Check sheet for the modelled part. Datum: model origin and axes. Units: mm. A direction names the side the tool comes from. Give positions to 0.01 mm unless a question says otherwise; leave off trailing zeros. Write each loop counter-clockwise with the first axis right and the second up, starting at its lowest first coordinate (ties: lowest second). Pieces come first, ordered by that corner, then holes. Notation, with made-up numbers: M -18,34 L 16,34 A6 cw 16,44 Z; hole C 29,-11.75 d6. An arc over 180 degrees is marked long. Write item = value, one per line. Start each with the question number.
1) Sectioned sample at C-C, the plane y = 1. Record the cut outline in (x, z) (3 decimals).
2) Gauge pin test, flat ends, axial feed: pin 1 (3.5 mm diameter, centred on x = 0, z = 0, fed in from -Y); pin 2 (2 mm diameter, centred on y = -4.5, z = -3.5, fed in from -X); pin 3 (1.6 mm diameter, centred on x = -11.5, z = 11.5, fed in from -Y); pin 4 (1.2 mm diameter, centred on x = -11.5, z = -11.5, fed in from +Y). Record the tip position at first contact, or that the pin passes through.
3) Sectioned sample at A-A, the plane y = 31. Record the cut outline in (x, z).
4) Draft check along X on faces 5 (the face through (6, 47, 16)), 6 (the face through (-2.003, 21.496, -0.631)), 7 (the face through (-3, 50, 3)), 8 (the face through (0, 25, 14.1)). Enter one of: pulls with the +X half, pulls with the -X half, needs draft (parallel to the pull), parting line crosses it, or undercut.
5) Scan lines: L1, parallel to Z at x = 0, y = 50.2; L2, parallel to Z at x = 0, y = 24.5; L3, parallel to Z at x = -11.5, y = 7.75 (3 decimals). Record each from-to range of solid material in increasing order.
6) Set-up check for faces 1 (the face through (-12.26, 7.6, -12.19)), 2 (the face through (11, 48, 11)), 3 (the face through (6, 51, 0)), 4 (the face through (-13, 49, -8.5)): record each of +Z, -Z, +X, -X, +Y, -Y from which the full face is reachable in a straight line by a thin tool's end or side.
from build123d import *

# Parameters (mm, degrees)
SKETCH1_W               = 28.2
SKETCH1_H               = 28.2
BOSS_EXTRUDE1_DEPTH     = 51
SKETCH2_R               = 11
BOSS_EXTRUDE2_DEPTH     = 2
M2_5_TAPPED_HOLE1_D     = 2.05
M2_5_TAPPED_HOLE1_DEPTH = 15
M2_5_TAPPED_HOLE1_TIP   = 0.615882135
FILLET1_R               = 3
SKETCH6_R               = 4
BOSS_EXTRUDE3_DEPTH     = 14
SKETCH7_R               = 4
BOSS_EXTRUDE4_DEPTH     = 7
M5_TAPPED_HOLE1_D       = 4.2
CHAMFER1_SIZE           = 0.2
SKETCH10_R              = 4.5
SKETCH10_R_2            = 4
CUT_EXTRUDE1_DEPTH      = 1
SKETCH11_W              = 12
SKETCH11_H              = 4
BOSS_EXTRUDE5_DEPTH     = 3
CUT_EXTRUDE2_DEPTH      = 3
CIRPATTERN1_COUNT       = 4
FILLET2_R               = 0.5


with BuildPart() as part:
    # Sketch1 → Boss-Extrude1 (new body)
    with BuildSketch(Plane(origin=(0, 0, 0), x_dir=(1, 0, 0), z_dir=(0, 1, 0))):
        Rectangle(SKETCH1_W, SKETCH1_H)
    extrude(amount=BOSS_EXTRUDE1_DEPTH)

    # Sketch2 → Boss-Extrude2 (add)
    with BuildSketch(Plane.XZ):
        Circle(SKETCH2_R)
    extrude(amount=BOSS_EXTRUDE2_DEPTH)

    # M2.5 Tapped Hole1
    with Locations(Plane(origin=(0, 0, 0), x_dir=(-1, 0, 0), z_dir=(0, -1, 0))):
        with Locations((11.5, -11.5), (-11.5, -11.5), (-11.5, 11.5), (11.5, 11.5)):
            Hole(M2_5_TAPPED_HOLE1_D / 2, depth=M2_5_TAPPED_HOLE1_DEPTH)
            with Locations((0, 0, -(M2_5_TAPPED_HOLE1_DEPTH + M2_5_TAPPED_HOLE1_TIP / 2))):  # 118° drill point
                Cone(0, M2_5_TAPPED_HOLE1_D / 2, M2_5_TAPPED_HOLE1_TIP, mode=Mode.SUBTRACT)

    # Fillet1
    fillet1_edges = [part.edges().sort_by_distance(p)[0] for p in [
        (14.1, 25.5, 14.1),
        (-14.1, 25.5, 14.1),
        (-14.1, 25.5, -14.1),
        (14.1, 25.5, -14.1),
    ]]
    fillet(fillet1_edges, radius=FILLET1_R)

    # Sketch6 → Boss-Extrude3 (add)
    with BuildSketch(Plane.XZ):
        Circle(SKETCH6_R)
    extrude(amount=BOSS_EXTRUDE3_DEPTH)

    # Sketch7 → Boss-Extrude4 (add)
    with BuildSketch(Plane(origin=(0, 51, 0), x_dir=(1, 0, 0), z_dir=(0, 1, 0))):
        Circle(SKETCH7_R)
    extrude(amount=BOSS_EXTRUDE4_DEPTH)

    # M5 Tapped Hole1 (through all)
    with Locations(Plane(origin=(0, 58, 0), x_dir=(1, 0, 0), z_dir=(0, 1, 0))):
        with Locations((0, 0)):
            Hole(M5_TAPPED_HOLE1_D / 2)

    # Chamfer1
    chamfer1_edges = [part.edges().sort_by_distance(p)[0] for p in [
        (-11, -2, 0),
        (-4, -14, 0),
        (-4, 58, 0),
    ]]
    chamfer(chamfer1_edges, length=CHAMFER1_SIZE)

    # Sketch10 → Cut-Extrude1 (cut)
    with BuildSketch(Plane(origin=(0, 51, 0), x_dir=(1, 0, 0), z_dir=(0, 1, 0))):
        Circle(SKETCH10_R)
        Circle(SKETCH10_R_2, mode=Mode.SUBTRACT)
    extrude(amount=-CUT_EXTRUDE1_DEPTH, mode=Mode.SUBTRACT)

    # Sketch11 → Boss-Extrude5 (add)
    with BuildSketch(Plane.XY.offset(14.1)):
        with Locations((0, 47)):
            Rectangle(SKETCH11_W, SKETCH11_H)
    extrude(amount=BOSS_EXTRUDE5_DEPTH)

    # Sketch12 → Cut-Extrude2 (cut)
    with BuildSketch(Plane(origin=(0, 51, 0), x_dir=(1, 0, 0), z_dir=(0, 1, 0))):
        with BuildLine():
            ThreePointArc((-11.5, 8.5), (-9.378679656, 9.378679656), (-8.5, 11.5))
            Line((-8.5, 11.5), (-8.5, 14.1))
            Line((-8.5, 14.1), (-11.1, 14.1))
            ThreePointArc((-11.1, 14.1), (-13.221320344, 13.221320344), (-14.1, 11.1))
            Line((-14.1, 11.1), (-14.1, 8.5))
            Line((-14.1, 8.5), (-11.5, 8.5))
        make_face()
    cut_extrude2 = extrude(amount=-CUT_EXTRUDE2_DEPTH, mode=Mode.SUBTRACT)

    # CirPattern1: Cut-Extrude2 ×4 about axis
    cirpattern1_axis = Axis((0, 0, 0), (0, 1, 0))
    for i in range(1, CIRPATTERN1_COUNT):
        add(cut_extrude2.rotate(cirpattern1_axis, i * 360 / CIRPATTERN1_COUNT), mode=Mode.SUBTRACT)

    # Fillet2
    fillet2_edges = [part.edges().sort_by_distance(p)[0] for p in [
        (-14.1, 51, 0),
        (-9.378679656, 51, -9.378679656),
        (-12.8, 51, -8.5),
        (-14.1, 48, -9.8),
        (-14.1, 49.5, -8.5),
        (-13.221320344, 48, -13.221320344),
        (-9.8, 48, -14.1),
        (-8.5, 49.5, -14.1),
        (-8.5, 51, -12.8),
        (0, 51, -14.1),
        (9.378679656, 51, -9.378679656),
        (8.5, 51, -12.8),
        (9.8, 48, -14.1),
        (8.5, 49.5, -14.1),
        (13.221320344, 48, -13.221320344),
        (14.1, 48, -9.8),
        (14.1, 49.5, -8.5),
        (12.8, 51, -8.5),
        (14.1, 51, 0),
        (9.378679656, 51, 9.378679656),
        (12.8, 51, 8.5),
        (14.1, 48, 9.8),
        (14.1, 49.5, 8.5),
        (13.221320344, 48, 13.221320344),
        (9.8, 48, 14.1),
        (8.5, 49.5, 14.1),
        (8.5, 51, 12.8),
        (0, 51, 14.1),
        (-9.378679656, 51, 9.378679656),
        (-8.5, 51, 12.8),
        (-9.8, 48, 14.1),
        (-8.5, 49.5, 14.1),
        (-13.221320344, 48, 13.221320344),
        (-14.1, 48, 9.8),
        (-14.1, 49.5, 8.5),
        (-12.8, 51, 8.5),
    ]]
    fillet(fillet2_edges, radius=FILLET2_R)


solid = part.part
Data:
q1.outline = M -14.1,-11.1 A3 ccw -11.1,-14.1 L 11.1,-14.1 A3 ccw 14.1,-11.1 L 14.1,11.1 A3 ccw 11.1,14.1 L -11.1,14.1 A3 ccw -14.1,11.1 Z; hole C -11.5,-11.5 d2.05; hole C -11.5,11.5 d2.05; hole C 0,0 d4.2; hole C 11.5,-11.5 d2.05; hole C 11.5,11.5 d2.05
q2.pin_1 = through
q2.pin_2 = -3.12
q2.pin_3 = 15.14
q2.pin_4 = 48
q3.outline = M -14.1,-11.1 A3 ccw -11.1,-14.1 L 11.1,-14.1 A3 ccw 14.1,-11.1 L 14.1,11.1 A3 ccw 11.1,14.1 L -11.1,14.1 A3 ccw -14.1,11.1 Z; hole C 0,0 d4.2
q4.face_5 = pulls with the +X half
q4.face_6 = undercut
q4.face_7 = undercut
q4.face_8 = needs draft
q5.L1 = -14.1 to -4.5, -4 to -2.1, 2.1 to 4, 4.5 to 14.1
q5.L2 = -14.1 to -2.1, 2.1 to 14.1
q5.L3 = -14.073 to -12.525, -10.475 to 10.475, 12.525 to 14.073
q6.face_1 = -Y
q6.face_2 = +Z, +X, +Y
q6.face_3 = +Y
q6.face_4 = -Z, -X, +Y
